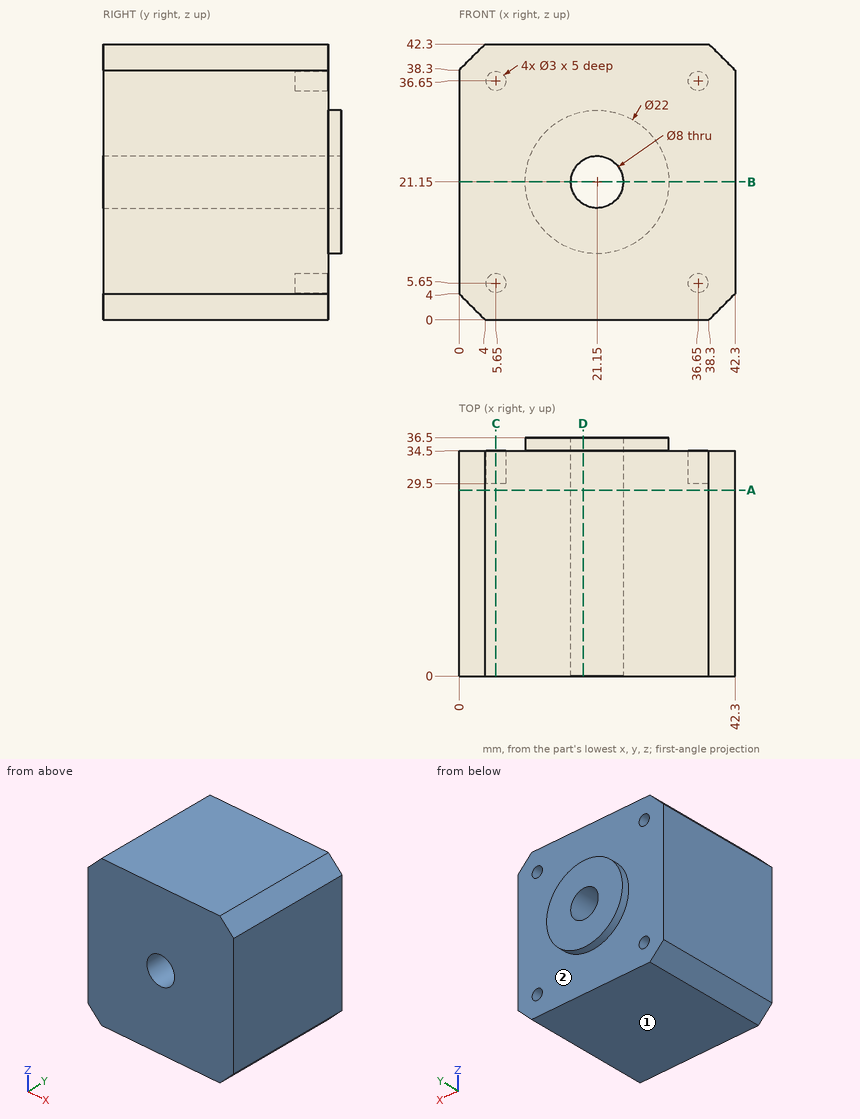
The drawing under review shows one solid part. Ordinate dimensions are in mm from its lowest x, y, z. A direction names the side the tool comes from. Round coordinates to 2 decimals unless told otherwise and drop trailing zeros. Order: outer loops, then holes, each group sorted by start corner. A loop starts at its lowest first (then second) coordinate and runs counter-clockwise, first axis right, second up. Notation, with made-up numbers: M 68.25,87.25 L 126.25,87.25 A26 cw 126.25,124.25 Z; hole C -23.5,34.5 d6. An arc over 180 degrees is marked long. Answer as CSV lines item,"result". Start each with the question number.
1) Wall thickness on line 1 along X through (y, z) = (32.45, 36.65); line 2 along Z through (x, y) = (5, 32): over which ranges is each line inside the solid? List them lowest first. Write a range as [from, to].
2) For pin 1 Ø2.5 at (x, z) = (37, 36.5) entering from +Y; pin 2 Ø6.5 at (x, z) = (21.15, 21.15) entering from -Y; pin 3 Ø1.8 at (x, z) = (5.65, 36.65) entering from +Y, all flat-tipped, find the tip position at first contact; note any pin that passes through.
3) Add section A-A (y = 28.5). Give the boundary of the cut face in (x, z).
4) Add section B-B (z = 21.15). Give the boundary of the cut face in (x, y), then the cut area to 3 significant figures.
5) Add section D-D (x = 19). Give the boundary of the cut face in (y, z).
6) Add section C-C (x = 5.65). Give the boundary of the cut face in (y, z), then the cut area to 3 significant figures.
7) Tool access review of the marked faces 1 and 2: name each direction out of +Z, -Z, +X, -X, +Y, -Y from which nothing blocks a thin tool from reaching the whole face with its end or side.
Resolved:
1,line 1,"[0, 4.15], [7.15, 35.15], [38.15, 42.3]"
1,line 2,"[0, 4.3], [7, 35.3], [38, 42.3]"
2,pin 1,"y = 34.5"
2,pin 2,"through"
2,pin 3,"y = 29.5"
3,outline,"M 0,4 L 4,0 L 38.3,0 L 42.3,4 L 42.3,38.3 L 38.3,42.3 L 4,42.3 L 0,38.3 Z; hole C 21.15,21.15 d8"
4,outline,"M 0,0 L 17.15,0 L 17.15,36.5 L 10.15,36.5 L 10.15,34.5 L 0,34.5 Z; M 25.15,0 L 42.3,0 L 42.3,34.5 L 32.15,34.5 L 32.15,36.5 L 25.15,36.5 Z"
4,area,"1,210 mm^2"
5,outline,"M 0,0 L 34.5,0 L 34.5,10.36 L 36.5,10.36 L 36.5,17.78 L 0,17.78 Z; M 0,24.52 L 36.5,24.52 L 36.5,31.94 L 34.5,31.94 L 34.5,42.3 L 0,42.3 Z"
6,outline,"M 0,0 L 34.5,0 L 34.5,4.15 L 29.5,4.15 L 29.5,7.15 L 34.5,7.15 L 34.5,35.15 L 29.5,35.15 L 29.5,38.15 L 34.5,38.15 L 34.5,42.3 L 0,42.3 Z"
6,area,"1,430 mm^2"
7,face 1,"-Z, +X, -X, +Y, -Y"
7,face 2,"+Y"
